Part model, mm, in its own coordinate system. Coordinates: 2 decimals unless noted, no trailing zeros. Write each loop counter-clockwise with the first axis right and the second up, starting at its lowest first coordinate (ties: lowest second). Pieces come first, ordered by that corner, then holes. Notation, with made-up numbers: M 37.25,67.5 L 46.25,67.5 A11 cw 46.25,76.5 Z; hole C 31,-27 d3. An arc over 180 degrees is marked long. Use a Markdown table: item, result. Add a question column.
Q1. Slice it at C-C on x = 8.5. Write the cut outline in (y, z).
Q2. Slice it at A-A on x = -8. Write the cut outline in (y, z), then the cut area to 3 significant figures.
Q3. Wall check: L1, parallel to X at y = -10.5, z = 2.5; L2, parallel to X at y = -9.5, z = 5; L3, parallel to Y at x = 8, z = 3.5. Give the ranges that are in metal, low to high. Write a range as from..to.
Q4. Slice it at B-B on y = 13. Write the cut outline in (x, z).
Q5. Slice it at D-D on z = 1.25. Write the cut outline in (x, y), then the cut area to 3 significant figures.
Q6. Mould opens along X. For faces 1 (the cylindrical face through (15.33, 18.41, 4.56)), 2 (the flat face through (-2, 19.84, 4)), 3 (the cylindrical face through (-3.352, 3.672, 4.437)) say: released by +X, released by -X, zero draft, split by the parting line, or undercut.
from build123d import *

# Parameters (mm, degrees)
SKETCH_1_W      = 38
SKETCH_1_H      = 38
SKETCH_1_R      = 2.5
SKETCH_1_R_2    = 3.05
EXTRUDE_1_DEPTH = 9
FILLET_1_R      = 5


with BuildPart() as part:
    # 草图1 → 凸台-拉伸1 (new body)
    with BuildSketch(Plane.XY):
        with Locations((-2.169799589, 0.839779006)):
            Rectangle(SKETCH_1_W, SKETCH_1_H)
        with Locations((8.830200411, 11.839779006)):
            Circle(SKETCH_1_R, mode=Mode.SUBTRACT)
        with Locations((8.830200411, -10.160220994)):
            Circle(SKETCH_1_R, mode=Mode.SUBTRACT)
        with Locations((-13.169799589, -10.160220994)):
            Circle(SKETCH_1_R, mode=Mode.SUBTRACT)
        with Locations((-6.169799589, 4.839779006)):
            Circle(SKETCH_1_R_2, mode=Mode.SUBTRACT)
    extrude(amount=EXTRUDE_1_DEPTH)

    # 圆角1
    fillet_1_edges = [part.edges().sort_by_distance(p)[0] for p in [
        (-21.169799589, 19.839779006, 4.5),
        (16.830200411, 19.839779006, 4.5),
        (16.830200411, -18.160220994, 4.5),
        (-21.169799589, -18.160220994, 4.5),
    ]]
    fillet(fillet_1_edges, radius=FILLET_1_R)


solid = part.part
Recorded:
| question | item | result |
|---|---|---|
| 1 | outline | M -18.16,0 L -12.64,0 L -12.64,9 L -18.16,9 Z; M -7.68,0 L 9.36,0 L 9.36,9 L -7.68,9 Z; M 14.32,0 L 19.84,0 L 19.84,9 L 14.32,9 Z |
| 2 | outline | M -18.16,0 L 2.4,0 L 2.4,9 L -18.16,9 Z; M 7.28,0 L 19.84,0 L 19.84,9 L 7.28,9 Z |
| 2 | area | 298 mm² |
| 3 | L1 | -21.17..-15.65, -10.69..6.35, 11.31..16.83 |
| 3 | L2 | -21.17..-15.58, -10.76..6.42, 11.24..16.83 |
| 3 | L3 | -18.16..-12.52, -7.8..9.48, 14.2..19.84 |
| 4 | outline | M -21.17,0 L 6.62,0 L 6.62,9 L -21.17,9 Z; M 11.04,0 L 16.83,0 L 16.83,9 L 11.04,9 Z |
| 5 | outline | M -21.17,-13.16 A5 ccw -16.17,-18.16 L 11.83,-18.16 A5 ccw 16.83,-13.16 L 16.83,14.84 A5 ccw 11.83,19.84 L -16.17,19.84 A5 ccw -21.17,14.84 Z; hole C -13.17,-10.16 d5; hole C -6.17,4.84 d6.1; hole C 8.83,-10.16 d5; hole C 8.83,11.84 d5 |
| 5 | area | 1,330 mm² |
| 6 | face 1 | released by +X |
| 6 | face 2 | zero draft |
| 6 | face 3 | undercut |
